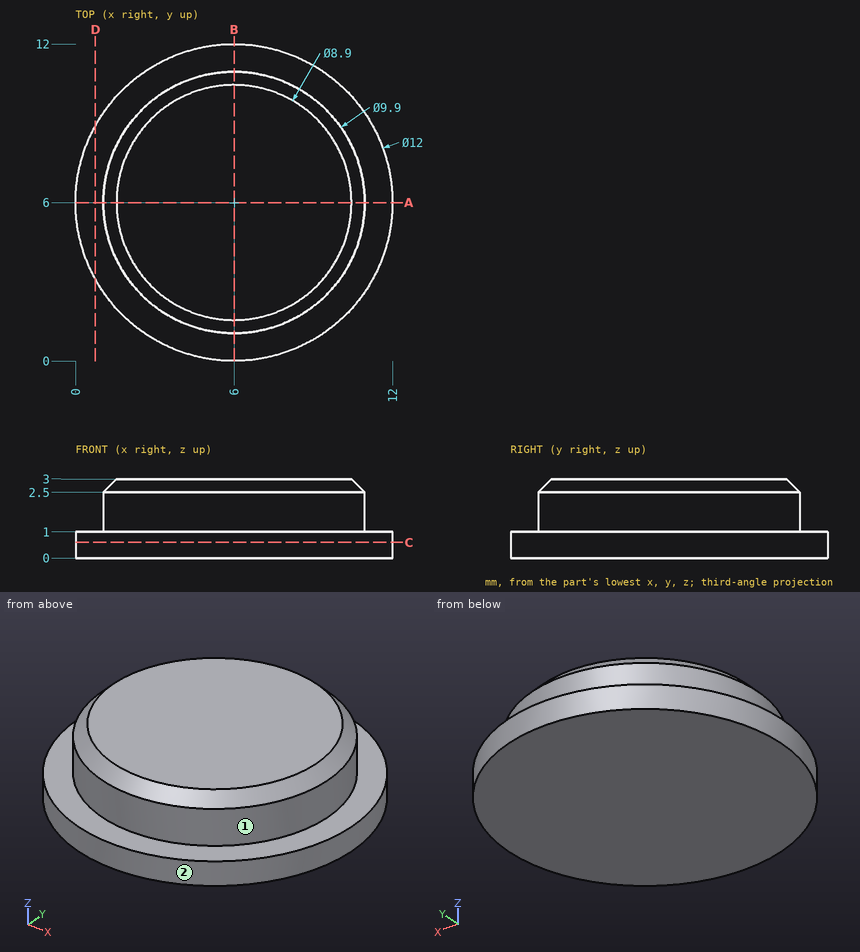
Input: dimensioned drawing with shaded views. Units: mm. Origin: part minimum x, y, z. A direction names the side the tool comes from. Round coordinates to 2 decimals unless told otherwise and drop trailing zeros. Loops run counter-clockwise (first coordinate to the right, second up) from the corner with the lowest first, then second, coordinate; pieces in that order, holes last. Notation, with made-up numbers: (0, 86) -> (48, 86) arc R23 ccw to (48, 102) -> close; hole circle Ø5 at (53, -24). An arc over 180 degrees is marked (long way). Answer as a JSON object with one key per item and string values. Group by question number.
Q1. Section query C-C (z = 0.6). Output: boundary loops of the cut face in (x, y), plus the area to 3 significant figures.
Q2. Section query A-A (y = 6). Output: boundary loops of the cut face in (x, z).
Q3. Contact query for flat-ended pins moving along their axis: P1, Ø1.5, axis at x = 10, z = 2.5, coming from the -Y side; P2, Ø1.5, axis at x = 4.5, z = 2, coming from the -Y side. Output: stop coordinate, or through.
Q4. Section query D-D (x = 0.75). Output: boundary loops of the cut face in (y, z), plus the area to 3 significant figures.
Q5. Ray query, line 1 (Z direction, x = 10, y = 2.75); line 2 (Y direction, x = 10, z = 0.65); line 3 (Y direction, x = 3.5, z = 2.6). Return the intervals inside material, ascending. Write a range as from..to.
Q6. Access query for the marked faces 1 and 2. Directions: +Z, -Z, +X, -X, +Y, -Y. A direction counts if a zero-diameter tool reaches every point of the face in a straight line with its end or side. Return the directions, or none.
Completed:
{
 "1": {"outline": "circle Ø12 at (6, 6)", "area": "113 mm²"},
 "2": {"outline": "(0, 0) -> (12, 0) -> (12, 1) -> (10.95, 1) -> (10.95, 2.5) -> (10.45, 3) -> (1.55, 3) -> (1.05, 2.5) -> (1.05, 1) -> (0, 1) -> close"},
 "3": {"P1": "y = 2.27", "P2": "y = 1.11"},
 "4": {"outline": "(3.1, 0) -> (8.9, 0) -> (8.9, 1) -> (3.1, 1) -> close", "area": "5.81 mm²"},
 "5": {"line 1": "0..1", "line 2": "1.53..10.47", "line 3": "1.84..10.16"},
 "6": {"face 1": "+Z", "face 2": "+Z, -Z"}
}
